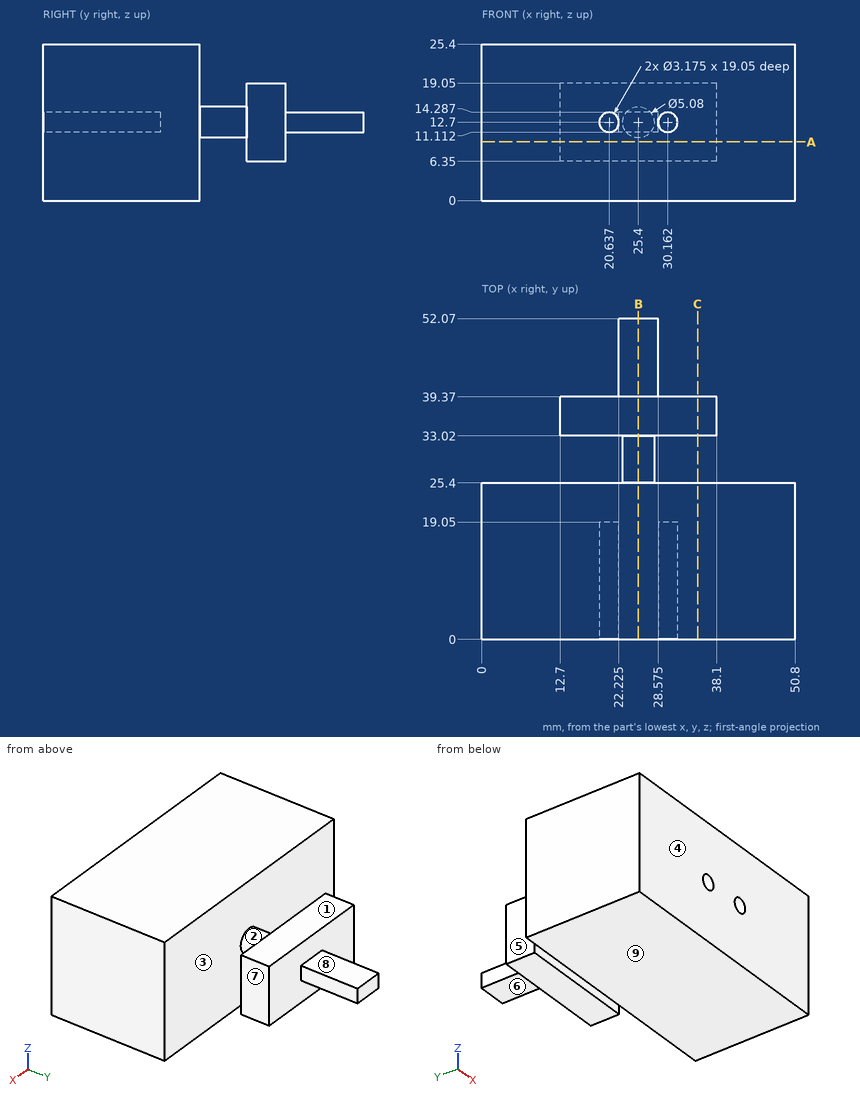
Here's the drawing with two shaded views (mm, measured from the low corner). I have some questions. A direction names the side the tool comes from. Round coordinates to 2 decimals unless told otherwise and drop trailing zeros. Loops run counter-clockwise (first coordinate to the right, second up) from the corner with the lowest first, then second, coordinate; pieces in that order, holes last. Notation, with made-up numbers: (21, -0.75) - (35, -0.75) arc R31 ccw to (35, 24.25) - close; hole circle Ø4 at (69, -11). An arc over 180 degrees is marked (long way). Use CSV: the item, a comma, the result in double quotes.
Item 1: If we section it at C-C on x = 35: List the corners of the cut face in (y, z) for me, then the cut area to 3 significant figures.
Here are the results:
outline,"(0, 0) - (25.4, 0) - (25.4, 25.4) - (0, 25.4) - close; (33.02, 6.35) - (39.37, 6.35) - (39.37, 19.05) - (33.02, 19.05) - close"
area,"726 mm²"
Item 2: Will these pins go through, and if not, where does the flat tip stop? pin 1 (5 mm diameter, centred on x = 26, y = 47, fed in from +Z); pin 2 (5 mm diameter, centred on x = 24.5, y = 35, fed in from +Z); pin 3 (5 mm diameter, centred on x = 34.5, y = 37.5, fed in from -Z).
Here are the results:
pin 1,"stops at z = 14.29"
pin 2,"stops at z = 19.05"
pin 3,"stops at z = 6.35"
Item 3: For the marked faces 5, 6, 7, 8 and 9, which set-ups out of +Z, -Z, +X, -X, +Y, -Y let a thin tool reach every point of the face, with its end or its side?
Here are the results:
face 5,"+Z, -Z, -X, +Y"
face 6,"-Z, +X, -X, +Y"
face 7,"+Z, -Z, +X, +Y"
face 8,"+Z, +X, -X, +Y"
face 9,"-Z, +X, -X, +Y, -Y"
Item 4: If we mould it in two halves opening along Y, with no side actions, what happens to the marked faces 1, 2, 3 and 4? For each: pulls with the +Y half, pulls with the -Y half, needs draft (parallel to the pull), parting line crosses it, or undercut.
Here are the results:
face 1,"needs draft"
face 2,"undercut"
face 3,"undercut"
face 4,"pulls with the -Y half"
Item 5: If we section it at B-B on x = 25.4: List the corners of the cut face in (y, z) for me.
Here are the results:
outline,"(0, 0) - (25.4, 0) - (25.4, 10.16) - (33.02, 10.16) - (33.02, 6.35) - (39.37, 6.35) - (39.37, 11.11) - (52.07, 11.11) - (52.07, 14.29) - (39.37, 14.29) - (39.37, 19.05) - (33.02, 19.05) - (33.02, 15.24) - (25.4, 15.24) - (25.4, 25.4) - (0, 25.4) - close"
Item 6: I need wall thicknesses on L1, parallel to Y at x = 31.5, z = 14; L2, parallel to Y at x = 3, z = 8; L3, parallel to X at y = 8, z = 13 (1 decimal). Which ranges of each line are inside material? Lowest first, please. Write a range as [from, to].
Here are the results:
L1,"y = [0, 25.4], [33.02, 39.37]"
L2,"y = [0, 25.4]"
L3,"x = [0, 19.1], [22.2, 28.6], [31.7, 50.8]"
Item 7: If we section it at A-A on z = 9.5: List the corners of the cut face in (x, y) for me, then the cut area to 3 significant figures.
Here are the results:
outline,"(0, 0) - (50.8, 0) - (50.8, 25.4) - (0, 25.4) - close; (12.7, 33.02) - (38.1, 33.02) - (38.1, 39.37) - (12.7, 39.37) - close"
area,"1,450 mm²"
